Autodesk Inventor part; units mm, degrees
ref_plane "YZ Plane" through (0, 0, 0) normal (1, 0, 0) x (0, 1, 0)
ref_plane "XZ Plane" through (0, 0, 0) normal (0, 1, 0) x (-1, 0, 0)
ref_plane "XY Plane" through (0, 0, 0) normal (0, 0, 1) x (1, 0, 0)
sketch "Sketch1" plane through (0, 0, 0) normal (0, 0, 1) x (1, 0, 0)
  line L0 (0, 0) -> (5.5, 0) construction
  line L1 (5.5, 0) -> (5.5, -2)
  line L2 (0, -8.6) -> (12.34, -8.6) construction
  line L3 (12.34, -8.6) -> (12.34, -5.5)
  line L4 (5.5, -2) -> (6.84, -2)
  line L5 (10.34, -5.5) -> (10.34, -8.6)
  line L6 (5.5, 0) -> (6.84, 0)
  arc A0 (10.34, -5.5) -> (6.84, -2) centre (6.84, -5.5) ccw
  arc A1 (12.34, -5.5) -> (6.84, 0) centre (6.84, -5.5) ccw
  line L7 (10.34, -8.6) -> (12.34, -8.6)
  line L8 (0, 0) -> (0, -8.6)
  dimension "d0" = 5.5
  dimension "d1" = 2
  dimension "d2" = 12.34
  dimension "d3" = 8.6
  dimension "d6" = 2
  dimension "d7" = 0
  dimension "d8" = 3.5
  dimension "d9" = 5.5
revolve "Revolution1" add sketch "Sketch1" angle 360 about axis through (0, 0, 0) along (0, -1, 0)
properties part number "BallBearingCup"
The model under review builds one solid part; all positions refer to its coordinate system, in mm. A direction names the side the tool comes from. Give positions to 0.01 mm unless a question says otherwise; leave off trailing zeros. Write each loop counter-clockwise with the first axis right and the second up, starting at its lowest first coordinate (ties: lowest second). Pieces come first, ordered by that corner, then holes. Notation, with made-up numbers: M 35,59.25 L 70,59.25 A37 cw 70,96.25 Z; hole C -34,10 d8. An arc over 180 degrees is marked long. One line per question, with ' | ' between items. Start each with the question number.
Item 1: We need section A-A on z = 0. Write out the cut boundary in (x, y).
Item 2: We need section B-B on x = 0. Write out the cut boundary in (y, z), plus the area to 3 significant figures.
Item 3: Draft analysis for pull direction Z (two halves, no side actions). For faces 3 (the cylindrical face through (-2.675, -7.028, 12.047)), 4 (the cylindrical face through (5.56, -7.07, 8.72)), 5 (the flat face through (-5, 0, 3)), state which applies: released by +Z, released by -Z, zero draft, split by the parting line, or undercut.
Item 4: For faces 1 (the flat face through (5.4, -8.6, -9.1)), 2 (the flat face through (-5, -2, 3)), list the 3-axis set-ups (+Z, -Z, +X, -X, +Y, -Y) from which the entire face can be reached by the end or side of a thin tool; tool diameter is ignored.
Item 5: We need section D-D on y = -1.25. Write out the cut boundary in (x, z).
Item 6: We need section C-C on y = -6.75. Write out the cut boundary in (x, z), plus the area to 3 significant figures.
Item 7: For pin 1 (1 mm diameter, centred on y = -4.5, z = -4, fed in from -X); pin 2 (2 mm diameter, centred on x = -9, z = -3, fed in from +Y); pin 3 (5 mm diameter, centred on y = -1.5, z = -3.5, fed in from +X); pin 4 (9 mm diameter, centred on x = 0, z = 0, fed in from -Y), all flat-tipped, find the tip position at first contact; note any pin that passes through.
Item 8: Wall thickness on line 1 (Y direction, x = -5.25, z = -3); line 2 (Z direction, x = -7, y = -3); line 3 (X direction, y = -6.5, z = -2.5): over which ranges is each line inside the solid? List them lowest first. Write a range as from..to.
Results found:
1) outline: M -12.34,-8.6 L -10.34,-8.6 L -10.34,-5.5 A3.5 cw -6.84,-2 L -5.5,-2 L -5.5,0 L -6.84,0 A5.5 ccw -12.34,-5.5 Z; M 5.5,-2 L 6.84,-2 A3.5 cw 10.34,-5.5 L 10.34,-8.6 L 12.34,-8.6 L 12.34,-5.5 A5.5 ccw 6.84,0 L 5.5,0 Z
2) outline: M -8.6,-12.34 L -5.5,-12.34 A5.5 ccw 0,-6.84 L 0,-5.5 L -2,-5.5 L -2,-6.84 A3.5 cw -5.5,-10.34 L -8.6,-10.34 Z; M -8.6,10.34 L -5.5,10.34 A3.5 cw -2,6.84 L -2,5.5 L 0,5.5 L 0,6.84 A5.5 ccw -5.5,12.34 L -8.6,12.34 Z | area: 46.0 mm2
3) face 3: split by the parting line | face 4: undercut | face 5: zero draft
4) face 1: +Z, -Z, +X, -X, -Y | face 2: -Y
5) outline: C 0,0 d20.66; hole C 0,0 d11
6) outline: C 0,0 d24.68; hole C 0,0 d20.68 | area: 143 mm2
7) pin 1: stops at x = -11.76 | pin 2: stops at y = -0.25 | pin 3: stops at x = 11.81 | pin 4: passes through
8) line 1: y = -2..0 | line 2: z = -9.42..-6.11, 6.11..9.42 | line 3: x = -12.08..-10.03, 10.03..12.08
